from build123d import *

# Parameters (mm, degrees)
SKETCH1_R                       = 2
SKETCH1_R_2                     = 3.125
SKETCH1_R_3                     = 1.7
BOSS_EXTRUDE1_DEPTH             = 10
FILLET2_R                       = 5
FILLET1_R                       = 2
SKETCH1_4_R                     = 3.125
CUT_EXTRUDE3_DEPTH              = 5.07
SKETCH1_7_R                     = 1.7
CUT_EXTRUDE6_DEPTH              = 10
CUT_EXTRUDE5_DEPTH              = 3
SKETCH1_5_R                     = 2
CUT_EXTRUDE4_DEPTH              = 2.48
SKETCH4_R                       = 1.5
CUT_EXTRUDE7_DEPTH              = 10
SKETCH5_R                       = 2.725
CUT_EXTRUDE8_DEPTH              = 2.8
BOSS_EXTRUDE2_DEPTH             = 10
BOSS_EXTRUDE3_DEPTH             = 35
FILLET13_R                      = 5
SKETCH10_W                      = 8
SKETCH10_H                      = 6
CUT_EXTRUDE12_DEPTH             = 40
FILLET14_R                      = 2
CUT_EXTRUDE17_DEPTH             = 35
TAP_DRILL_FOR_M3X0_5_TAP1_D     = 2.5
TAP_DRILL_FOR_M3X0_5_TAP1_DEPTH = 4.248924226
TAP_DRILL_FOR_M3X0_5_TAP1_TIP   = 0.751075774
SKETCH23_2_R                    = 3.25
BOSS_EXTRUDE7_DEPTH             = 2
FILLET16_R                      = 4
SKETCH23_R                      = 3.25
CUT_EXTRUDE20_DEPTH             = 10
CUT_EXTRUDE20_DEPTH_BACK        = 4


with BuildPart() as part:
    # Sketch1 → Boss-Extrude1 (new body)
    with BuildSketch(Plane(origin=(0, 0, 0), x_dir=(1, 0, 0), z_dir=(0, 1, 0))):
        with BuildLine():
            ThreePointArc((-11.409245094, 8.977987014), (-9.849239736, 9.28), (-8.289234378, 8.977987014))
            ThreePointArc((-8.289234378, 8.977987014), (-5.835653376, 8.254222737), (-3.289234378, 8.01))
            Line((-3.289234378, 8.01), (38.12, 8.01))
            Line((38.12, 8.01), (38.12, -3.81))
            Line((38.12, -3.81), (28.478275237, -3.81))
            Line((28.478275237, -3.81), (26.178275237, 0))
            Line((26.178275237, 0), (-26.178275237, 0))
            Line((-26.178275237, 0), (-28.478275237, -3.81))
            Line((-28.478275237, -3.81), (-38.12, -3.81))
            Line((-38.12, -3.81), (-38.12, 8.01))
            Line((-38.12, 8.01), (-16.409245094, 8.01))
            ThreePointArc((-16.409245094, 8.01), (-13.862826096, 8.254222737), (-11.409245094, 8.977987014))
        make_face()
        with Locations((22, 4.005)):
            Circle(SKETCH1_R, mode=Mode.SUBTRACT)
        with Locations((-22, 4.005)):
            Circle(SKETCH1_R, mode=Mode.SUBTRACT)
        with Locations((-32.12, 1.98)):
            Circle(SKETCH1_R_2, mode=Mode.SUBTRACT)
        with Locations((32.12, 1.98)):
            Circle(SKETCH1_R_2, mode=Mode.SUBTRACT)
        with Locations((-9.849239736, 5.1)):
            Circle(SKETCH1_R_3, mode=Mode.SUBTRACT)
        with BuildLine():
            ThreePointArc((11.912105026, 2.53), (14.127105026, 4.745), (11.912105026, 6.96))
            Line((11.912105026, 6.96), (5.992105026, 6.96))
            ThreePointArc((5.992105026, 6.96), (3.777105026, 4.745), (5.992105026, 2.53))
            Line((5.992105026, 2.53), (11.912105026, 2.53))
        make_face(mode=Mode.SUBTRACT)
        with Locations((-22, 4.005)):
            Circle(SKETCH1_R)
        with Locations((-9.849239736, 5.1)):
            Circle(SKETCH1_R_3)
        with Locations((-32.12, 1.98)):
            Circle(SKETCH1_R_2)
        with BuildLine():
            Line((5.992105026, 2.53), (11.912105026, 2.53))
            ThreePointArc((11.912105026, 2.53), (14.127105026, 4.745), (11.912105026, 6.96))
            Line((11.912105026, 6.96), (5.992105026, 6.96))
            ThreePointArc((5.992105026, 6.96), (3.777105026, 4.745), (5.992105026, 2.53))
        make_face()
        with Locations((22, 4.005)):
            Circle(SKETCH1_R)
        with Locations((32.12, 1.98)):
            Circle(SKETCH1_R_2)
    extrude(amount=-BOSS_EXTRUDE1_DEPTH)

    # Fillet2
    fillet2_edges = [part.edges().sort_by_distance(p)[0] for p in [
        (28.478275237, -5, 3.81),
        (-28.478275237, -5, 3.81),
    ]]
    fillet(fillet2_edges, radius=FILLET2_R)

    # Fillet1
    fillet1_edges = [part.edges().sort_by_distance(p)[0] for p in [
        (26.178275237, -5, 0),
        (-26.178275237, -5, 0),
    ]]
    fillet(fillet1_edges, radius=FILLET1_R)

    # Sketch1_4 → Cut-Extrude3 (cut)
    with BuildSketch(Plane(origin=(0, 0, 0), x_dir=(1, 0, 0), z_dir=(0, 1, 0))):
        with Locations(Location((32.12, 1.98, 0), (0, 0, 270))):
            Circle(SKETCH1_4_R)
        with Locations(Location((-32.12, 1.98, 0), (0, 0, 270))):
            Circle(SKETCH1_4_R)
    extrude(amount=-CUT_EXTRUDE3_DEPTH, mode=Mode.SUBTRACT)

    # Sketch1_7 → Cut-Extrude6 (cut)
    with BuildSketch(Plane(origin=(0, 0, 0), x_dir=(1, 0, 0), z_dir=(0, 1, 0))):
        with Locations(Location((-9.849239736, 5.1, 0), (0, 0, 270))):
            Circle(SKETCH1_7_R)
    extrude(amount=-CUT_EXTRUDE6_DEPTH, mode=Mode.SUBTRACT)

    # Sketch1_6 → Cut-Extrude5 (cut)
    with BuildSketch(Plane(origin=(0, 0, 0), x_dir=(1, 0, 0), z_dir=(0, 1, 0))):
        with BuildLine():
            Line((5.992105026, 2.53), (11.912105026, 2.53))
            ThreePointArc((11.912105026, 2.53), (14.127105026, 4.745), (11.912105026, 6.96))
            Line((11.912105026, 6.96), (5.992105026, 6.96))
            ThreePointArc((5.992105026, 6.96), (3.777105026, 4.745), (5.992105026, 2.53))
        make_face()
    extrude(amount=-CUT_EXTRUDE5_DEPTH, mode=Mode.SUBTRACT)

    # Sketch1_5 → Cut-Extrude4 (cut)
    with BuildSketch(Plane(origin=(0, 0, 0), x_dir=(1, 0, 0), z_dir=(0, 1, 0))):
        with Locations(Location((-22, 4.005, 0), (0, 0, 270))):
            Circle(SKETCH1_5_R)
        with Locations(Location((22, 4.005, 0), (0, 0, 270))):
            Circle(SKETCH1_5_R)
    extrude(amount=-CUT_EXTRUDE4_DEPTH, mode=Mode.SUBTRACT)

    # Sketch4 → Cut-Extrude7 (cut)
    with BuildSketch(Plane(origin=(0, 0, 0), x_dir=(1, 0, 0), z_dir=(0, 1, 0))):
        with Locations(Location((-22, 4.005, 0), (0, 0, 270))):
            Circle(SKETCH4_R)
        with Locations(Location((22, 4.005, 0), (0, 0, 270))):
            Circle(SKETCH4_R)
    extrude(amount=-CUT_EXTRUDE7_DEPTH, mode=Mode.SUBTRACT)

    # Sketch5 → Cut-Extrude8 (cut)
    with BuildSketch(Plane.XZ.offset(10)):
        with Locations(Location((22, -4.005, 0), (0, 0, 270))):
            Circle(SKETCH5_R)
        with Locations(Location((-22, -4.005, 0), (0, 0, 90))):
            Circle(SKETCH5_R)
    extrude(amount=-CUT_EXTRUDE8_DEPTH, mode=Mode.SUBTRACT)

    # Sketch6 → Boss-Extrude2 (add)
    with BuildSketch(Plane(origin=(0, 0, 0), x_dir=(1, 0, 0), z_dir=(0, 1, 0))):
        with BuildLine():
            Line((-38.12, 8.01), (-38.12, 18.01))
            Line((-38.12, 18.01), (38.12, 18.01))
            Line((38.12, 18.01), (38.12, 8.01))
            Line((38.12, 8.01), (-3.289234378, 8.01))
            ThreePointArc((-3.289234378, 8.01), (-5.835653376, 8.254222737), (-8.289234378, 8.977987014))
            ThreePointArc((-8.289234378, 8.977987014), (-9.849239736, 9.28), (-11.409245094, 8.977987014))
            ThreePointArc((-11.409245094, 8.977987014), (-13.862826096, 8.254222737), (-16.409245094, 8.01))
            Line((-16.409245094, 8.01), (-38.12, 8.01))
        make_face()
    extrude(amount=-BOSS_EXTRUDE2_DEPTH)

    # Sketch8 → Boss-Extrude3 (add)
    with BuildSketch(Plane.XZ.offset(10)):
        with BuildLine():
            Line((18.950546011, 0), (-18.950546011, 0))
            Line((-18.950546011, 0), (-18.950546011, -4.005))
            ThreePointArc((-18.950546011, -4.005), (-22, -7.054453989), (-25.049453989, -4.005))
            Line((-25.049453989, -4.005), (-25.049453989, 0))
            ThreePointArc((-25.049453989, 0), (-26.032503369, 0.25827272), (-26.761657912, 0.966386084))
            Line((-26.761657912, 0.966386084), (-27.019818549, 1.394034791))
            ThreePointArc((-27.019818549, 1.394034791), (-28.842704905, 3.164318199), (-31.300328355, 3.81))
            Line((-31.300328355, 3.81), (-38.12, 3.81))
            Line((-38.12, 3.81), (-38.12, -18.01))
            Line((-38.12, -18.01), (38.12, -18.01))
            Line((38.12, -18.01), (38.12, 3.81))
            Line((38.12, 3.81), (31.300328355, 3.81))
            ThreePointArc((31.300328355, 3.81), (28.842704905, 3.164318199), (27.019818549, 1.394034791))
            Line((27.019818549, 1.394034791), (26.761657912, 0.966386084))
            ThreePointArc((26.761657912, 0.966386084), (26.032503369, 0.25827272), (25.049453989, 0))
            Line((25.049453989, 0), (25.049453989, -4.005))
            ThreePointArc((25.049453989, -4.005), (22, -7.054453989), (18.950546011, -4.005))
            Line((18.950546011, -4.005), (18.950546011, 0))
        make_face()
    extrude(amount=BOSS_EXTRUDE3_DEPTH)

    # Fillet13
    fillet13_edges = [part.edges().sort_by_distance(p)[0] for p in [
        (-38.12, -22.5, -18.01),
    ]]
    fillet(fillet13_edges, radius=FILLET13_R)

    # Sketch10 → Cut-Extrude12 (cut)
    with BuildSketch(Plane(origin=(38.12, 0, 0), x_dir=(0, 0, -1), z_dir=(1, 0, 0))):
        with Locations((12.01, -3)):
            Rectangle(SKETCH10_W, SKETCH10_H)
    extrude(amount=-CUT_EXTRUDE12_DEPTH, mode=Mode.SUBTRACT)

    # Fillet14
    fillet14_edges = [part.edges().sort_by_distance(p)[0] for p in [
        (-1.88, -3, -16.01),
        (18.12, -6, -16.01),
        (-1.88, -3, -8.01),
    ]]
    fillet(fillet14_edges, radius=FILLET14_R)

    # Sketch18 → Cut-Extrude17 (cut)
    with BuildSketch(Plane.XZ.offset(45)):
        Polygon((-10, 0), (-10, -1.75), (-15, -1.75), (-15, -8.75), (15, -8.75), (15, -1.75), (10, -1.75), (10, 0), align=None)
    extrude(amount=-CUT_EXTRUDE17_DEPTH, mode=Mode.SUBTRACT)

    # Tap Drill for M3x0.5 Tap1
    with Locations(Plane.XY.offset(-8.75)):
        with Locations((0, -28), (0, -18)):
            Hole(TAP_DRILL_FOR_M3X0_5_TAP1_D / 2, depth=TAP_DRILL_FOR_M3X0_5_TAP1_DEPTH)
            with Locations((0, 0, -(TAP_DRILL_FOR_M3X0_5_TAP1_DEPTH + TAP_DRILL_FOR_M3X0_5_TAP1_TIP / 2))):  # 118° drill point
                Cone(0, TAP_DRILL_FOR_M3X0_5_TAP1_D / 2, TAP_DRILL_FOR_M3X0_5_TAP1_TIP, mode=Mode.SUBTRACT)

    # Sketch23_2 → Boss-Extrude7 (add)
    with BuildSketch(Plane.XZ.offset(10)):
        with Locations((-9.849239736, -5.1)):
            Circle(SKETCH23_2_R)
    extrude(amount=-BOSS_EXTRUDE7_DEPTH)

    # Fillet16
    fillet16_edges = [part.edges().sort_by_distance(p)[0] for p in [
        (-10, -10, -0.875),
        (-15, -10, -5.25),
        (15, -10, -5.25),
        (10, -10, -0.875),
    ]]
    fillet(fillet16_edges, radius=FILLET16_R)

    # Sketch23 → Cut-Extrude20 (cut, two sides)
    with BuildSketch(Plane.XZ.offset(10)) as cut_extrude20_sk:
        with Locations(Location((-9.849239736, -5.1, 0), (0, 0, 110.737075226))):
            Circle(SKETCH23_R)
    extrude(amount=CUT_EXTRUDE20_DEPTH, mode=Mode.SUBTRACT)
    extrude(cut_extrude20_sk.sketch, amount=-CUT_EXTRUDE20_DEPTH_BACK, mode=Mode.SUBTRACT)


solid = part.part
Could you check a few things on this model? Use its own coordinates, in mm. A direction names the side the tool comes from. Coordinates: 2 decimals unless noted, no trailing zeros. Order: outer loops, then holes, each group sorted by start corner. A loop starts at its lowest first (then second) coordinate and runs counter-clockwise, first axis right, second up.
Q1. Will these pins go through, and if not, where does the flat tip stop? pin 1 (2.5 mm diameter, centred on x = -0.5, z = -4, fed in from -Y); pin 2 (2 mm diameter, centred on x = -8.5, z = -6, fed in from -Y); pin 3 (3 mm diameter, centred on x = 11.5, y = -25, fed in from +Z).
Q2. Please list where these lines run through material, in increasing order: L1, parallel to Y at x = 0, z = -9.9; L2, parallel to Z at x = -22, y = -8; L3, parallel to X at y = -35, z = -0.25.
Q3. Suppose I cut it at B-B on x = -32.12. Please give me the cut outline in (y, z) (3 decimals), and give its area (3 significant figures).
Q4. Which directions (+Z, -Z, +X, -X, +Y, -Y) give clear straight access to the entire face, cutting with the end or side of a thin tool? Please do faces 1 (the flat face through (-18.951, -27, -2)), 2 (the cylindrical face through (13.797, -11.141, -5.201)), 3 (the flat face through (18, -6, -11)), 4 (the cylindrical face through (-29.02, -2.5, -2.39)).
Q5. Suppose I cut it at A-A on x = 22. Please give me the cut outline in (y, z) (3 decimals), and give its area (3 significant figures).
Q6. Suppose I cut it at C-C on y = -16. Please give me the cut outline in (x, z) (3 decimals).
Answer:
1. pin 1: stops at y = -10
1. pin 2: stops at y = -6
1. pin 3: stops at z = 0
2. L1: y = -45 to -29.25, -26.75 to -19.25, -16.75 to -6
2. L2: z = -18.01 to -6.73, -1.28 to 0
2. L3: x = -38.12 to -25.05, -18.95 to -10, 10 to 18.95, 25.05 to 38.12
3. outline: (-45, -18.01) - (0, -18.01) - (0, -5.105) - (-5.07, -5.105) - (-5.07, 1.145) - (0, 1.145) - (0, 3.81) - (-45, 3.81) - close
3. area: 950 mm2
4. face 1: +Z, -Y
4. face 2: -Y
4. face 3: +X, +Y
4. face 4: +Y
5. outline: (-45, -18.01) - (0, -18.01) - (0, -16.01) - (-4, -16.01) arc R2 cw to (-6, -14.01) - (-6, -8.01) - (0, -8.01) - (0, -6.005) - (-2.48, -6.005) - (-2.48, -5.505) - (-7.2, -5.505) - (-7.2, -6.73) - (-10, -6.73) - (-10, -7.054) - (-45, -7.054) - close; (-10, -1.28) - (-7.2, -1.28) - (-7.2, -2.505) - (-2.48, -2.505) - (-2.48, -2.005) - (0, -2.005) - (0, 0) - (-10, 0) - close
5. area: 477 mm2
6. outline: (-38.12, -13.01) arc R5 ccw to (-33.12, -18.01) - (38.12, -18.01) - (38.12, 3.81) - (31.3, 3.81) arc R5 ccw to (27.02, 1.394) - (26.762, 0.966) arc R2 cw to (25.049, 0) - (25.049, -4.005) arc R3.049 cw to (18.951, -4.005) - (18.951, 0) - (10, 0) - (10, -1.75) - (15, -1.75) - (15, -8.75) - (-15, -8.75) - (-15, -1.75) - (-10, -1.75) - (-10, 0) - (-18.951, 0) - (-18.951, -4.005) arc R3.049 cw to (-25.049, -4.005) - (-25.049, 0) arc R2 cw to (-26.762, 0.966) - (-27.02, 1.394) arc R5 ccw to (-31.3, 3.81) - (-38.12, 3.81) - close
